from build123d import *

# Parameters (mm, degrees)
F0_R     = 45
F1_DEPTH = 115
F2_R     = 22.5
F3_DEPTH = 24
F4_SIZE2 = 114.99999
F4_SIZE  = 19.99999


# Not quite as in the source:
# - a fillet or chamfer is up to 0.001 mm smaller than in the source, because OpenCascade refuses the exact size


with BuildPart() as f1:
    # F0 (on Top) → F1 (new body)
    with BuildSketch(Plane.XY):
        Circle(F0_R)
    extrude(amount=F1_DEPTH)

    # F2 (on face) → F3 (join)
    with BuildSketch(Plane(origin=(0, 0, 0), x_dir=(1, 0, 0), z_dir=(0, 0, -1))):
        Circle(F2_R)
    extrude(amount=F3_DEPTH)

    # F4 (size 20 and 115 in the source; OpenCascade refuses exactly that, so slightly less here)
    f4_edges = [f1.edges().sort_by_distance(p)[0] for p in [
        (-45, 0, 0),
    ]]
    f4_side = f1.faces().sort_by_distance((-43.727208, 0, 0))[0]
    chamfer(f4_edges, length=F4_SIZE, length2=F4_SIZE2, reference=f4_side)


solid = f1.part
The listing builds one solid part. Answer for the finished solid, in the listing's coordinates (mm). Coordinates: 2 decimals unless noted, no trailing zeros. Write each loop counter-clockwise with the first axis right and the second up, starting at its lowest first coordinate (ties: lowest second). Pieces come first, ordered by that corner, then holes. Notation, with made-up numbers: (-24.5, -39.5) - (-7.5, -39.5) arc R16 ccw to (-7.5, -18.5) - close; hole circle Ø2 at (-7, -1). An arc over 180 degrees is marked (long way). Return JSON: item names as keys, results as strings.
1. Consider line 1 along X through (y, z) = (34, 77.5); line 2 along X through (y, z) = (21.5, 22); line 3 along Y through (x, z) = (13.5, 91.5). Determine where each line is inside the solid, lowest interval first.
Final values:
{"line 1": "-18.02 to 18.02", "line 2": "-19.2 to 19.2", "line 3": "-38.62 to 38.62"}
2. For a pull along Z with two mould halves and no side action, classify faces 1 (the face through (10.382, 19.961, -11.832)), 2 (the face through (-1, 1, 115)), 3 (the face through (0, 0, -24)) as +Z half, -Z half, draft (parallel to the pull), parting line (faces both ways), or undercut.
Final values:
{"face 1": "draft", "face 2": "+Z half", "face 3": "-Z half"}
3. The part is cut by section C-C on z = -3. Determine the outline of the cut face in (x, y).
Final values:
{"outline": "circle Ø45 at (0, 0)"}
4. Each of these flat-tipped pins is pushed along its axis until it touches: pin 1 Ø3 at (x, z) = (-24, 72) entering from +Y; pin 2 Ø6 at (x, z) = (-19, 71.5) entering from +Y; pin 3 Ø2 at (y, z) = (-25, 36) entering from +X. Where does it stop, or does it pass through?
Final values:
{"pin 1": "y = 30.07", "pin 2": "y = 33.96", "pin 3": "x = 20.06"}
5. The part is cut by section D-D on z = 11. Determine the outline of the cut face in (x, y).
Final values:
{"outline": "circle Ø53.83 at (0, 0)"}
